```python
from build123d import *

# Parameters (mm, degrees)
BASE_EXTRUDE_DEPTH = 31.75
FILLET1_R          = 19.05


with BuildPart() as part:
    # Sketch5 → Base-Extrude (new, symmetric)
    with BuildSketch(Plane.ZY.offset(-254)):
        with BuildLine():
            ThreePointArc((9.918396921, -78.230607992), (-44.703978299, -33.86975469), (-91.248408889, -86.643850244))
            ThreePointArc((-91.248408889, -86.643850244), (-78.432247724, -229.591476611), (-52.225916685, -370.69961275))
            ThreePointArc((-52.225916685, -370.69961275), (-17.988619307, -396.10195786), (12.760925504, -366.573375727))
            ThreePointArc((12.760925504, -366.573375727), (19.549821807, -222.321054799), (9.918396921, -78.230607992))
        make_face()
    extrude(amount=BASE_EXTRUDE_DEPTH, both=True)

    # Fillet1
    fillet1_edges = [part.edges().sort_by_distance(p)[0] for p in [
        (222.25, -229.591476611, -78.432247724),
        (222.25, -396.10195786, -17.988619307),
        (222.25, -222.321054799, 19.549821807),
        (285.75, -396.10195786, -17.988619307),
        (285.75, -229.591476611, -78.432247724),
        (285.75, -33.86975469, -44.703978299),
        (285.75, -222.321054799, 19.549821807),
        (222.25, -33.86975469, -44.703978299),
    ]]
    fillet(fillet1_edges, radius=FILLET1_R)


solid = part.part
```
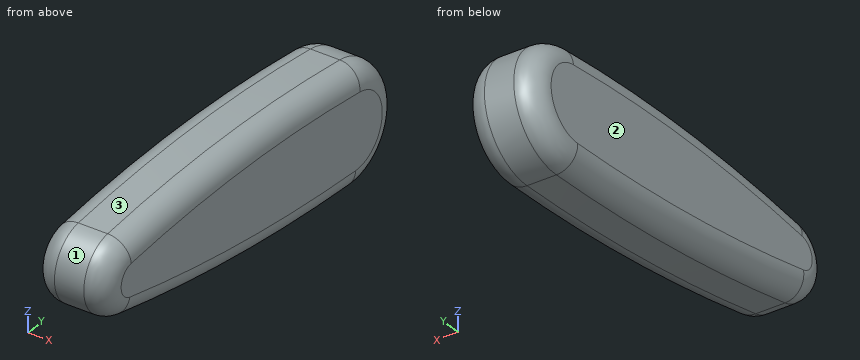
The model under review builds one solid part; all positions refer to its coordinate system, in mm. Face numbers are marked on the shaded views. Round coordinates to 2 decimals unless told otherwise and drop trailing zeros. Write each loop counter-clockwise with the first axis right and the second up, starting at its lowest first coordinate (ties: lowest second). Pieces come first, ordered by that corner, then holes. Notation, with made-up numbers: (25.5, 10) - (44.5, 10) arc R27 ccw to (44.5, 40) - close; hole circle Ø5 at (17.5, 32.5). An arc over 180 degrees is marked (long way). Answer as CSV lines item,"result". Start each with the question number.
(1) For pin 1 Ø12 at (x, z) = (270.5, -56.5) entering from +Y; pin 2 Ø1.5 at (y, z) = (-354.5, -58) entering from +X; pin 3 Ø1 at (x, z) = (252, -23.5) entering from +Y; pin 4 Ø6 at (x, y) = (253, -108) entering from +Z, all flat-tipped, find the tip position at first contact; note any pin that passes through.
(2) We need section A-A on x = 250. State the section outline as (y, z) points (3 decimals).
(3) Draft analysis for pull direction Y (two halves, no side actions). For the marked faces 1, 2 and 3, state which applies: pulls with the +Y half, pulls with the -Y half, needs draft (parallel to the pull), parting line crosses it, or undercut.
(4) To check wall thickness, follow line 1 (X direction, y = -128.5, z = -81); line 2 (Z direction, x = 265, y = -273); line 3 (Y direction, x = 270, z = -26). State the ranges of each line that lie inside material, in increasing order.
Worked answers:
1,pin 1,"y = -34.84"
1,pin 2,"through"
1,pin 3,"y = -36.45"
1,pin 4,"z = 13.56"
2,outline,"(-370.7, -52.226) arc R1524 ccw to (-86.644, -91.248) arc R50.8 ccw to (-78.231, 9.918) arc R1270 ccw to (-366.573, 12.761) arc R33.02 ccw to start"
3,face 1,"pulls with the -Y half"
3,face 2,"needs draft"
3,face 3,"parting line crosses it"
4,line 1,"225.87 to 282.13"
4,line 2,"-71.83 to 19.04"
4,line 3,"-395.34 to -36.11"
